```python
from build123d import *

# Parameters (mm, degrees)
SKETCH1_R           = 11.15
BOSS_EXTRUDE1_DEPTH = 15
FILLET3_R           = 0.8


with BuildPart() as part:
    # Sketch1 → Boss-Extrude1 (new body)
    with BuildSketch(Plane(origin=(0, 0, 0), x_dir=(1, 0, 0), z_dir=(0, 1, 0))):
        Polygon((0, 17.15), (2.145893606, 13.548639006), (5.299641454, 16.310619254), (6.227625801, 12.222403821), (10.080517077, 13.874641454), (9.699754592, 9.699754592), (13.874641454, 10.080517077), (12.222403821, 6.227625801), (16.310619254, 5.299641454), (13.548639006, 2.145893606), (17.15, 0), (13.548639006, -2.145893606), (16.310619254, -5.299641454), (12.222403821, -6.227625801), (13.874641454, -10.080517077), (9.699754592, -9.699754592), (10.080517077, -13.874641454), (6.227625801, -12.222403821), (5.299641454, -16.310619254), (2.145893606, -13.548639006), (0, -17.15), (-2.145893606, -13.548639006), (-5.299641454, -16.310619254), (-6.227625801, -12.222403821), (-10.080517077, -13.874641454), (-9.699754592, -9.699754592), (-13.874641454, -10.080517077), (-12.222403821, -6.227625801), (-16.310619254, -5.299641454), (-13.548639006, -2.145893606), (-17.15, 0), (-13.548639006, 2.145893606), (-16.310619254, 5.299641454), (-12.222403821, 6.227625801), (-13.874641454, 10.080517077), (-9.699754592, 9.699754592), (-10.080517077, 13.874641454), (-6.227625801, 12.222403821), (-5.299641454, 16.310619254), (-2.145893606, 13.548639006), align=None)
        Circle(SKETCH1_R, mode=Mode.SUBTRACT)
    extrude(amount=BOSS_EXTRUDE1_DEPTH)

    # Fillet3
    fillet3_edges = [part.edges().sort_by_distance(p)[0] for p in [
        (0, 7.5, -17.15),
        (5.299641454, 7.5, -16.310619254),
        (10.080517077, 7.5, -13.874641454),
        (13.874641454, 7.5, -10.080517077),
        (16.310619254, 7.5, -5.299641454),
        (17.15, 7.5, 0),
        (16.310619254, 7.5, 5.299641454),
        (13.874641454, 7.5, 10.080517077),
        (10.080517077, 7.5, 13.874641454),
        (5.299641454, 7.5, 16.310619254),
        (0, 7.5, 17.15),
        (-5.299641454, 7.5, 16.310619254),
        (-10.080517077, 7.5, 13.874641454),
        (-13.874641454, 7.5, 10.080517077),
        (-16.310619254, 7.5, 5.299641454),
        (-17.15, 7.5, 0),
        (-16.310619254, 7.5, -5.299641454),
        (-13.874641454, 7.5, -10.080517077),
        (-10.080517077, 7.5, -13.874641454),
        (-5.299641454, 7.5, -16.310619254),
    ]]
    fillet(fillet3_edges, radius=FILLET3_R)


solid = part.part
```
Geometry check sheet. Reference: the model listing, model coordinates, mm. A direction names the side the tool comes from. Give positions to 0.01 mm unless a question says otherwise; leave off trailing zeros. Write each loop counter-clockwise with the first axis right and the second up, starting at its lowest first coordinate (ties: lowest second). Pieces come first, ordered by that corner, then holes.
1) Access from +Z, -Z, +X, -X, +Y, -Y to the whole of each face (thin tool, end or side, straight path). Record for faces 5 (the flat face through (-14.8, 7.4, -1.4)), 6 (the flat face through (-1.4, 7.4, 14.8)), 7 (the flat face through (5.91, 7.4, -13.63)), 8 (the flat face through (14.8, 7.4, -1.4)).
2) Section check A-A, the plane z = 0. Record the boundary of the cut face in (x, y), and give its area (3 significant figures).
3) Gauge pin test, flat ends, axial feed: pin 1 (1 mm diameter, centred on y = 12.5, z = 3.5, fed in from -X); pin 2 (6 mm diameter, centred on y = 10, z = -9.5, fed in from -X); pin 3 (6 mm diameter, centred on y = 1.5, z = 3, fed in from +X); pin 4 (2 mm diameter, centred on y = 7, z = 9.5, fed in from +X). Record the tip position at first contact, or that the pin passes through.
4) Release check for a two-part mould opening along X. For faces 1 (the flat face through (-14.5, 7.4, 3.23)), 2 (the cylindrical face through (0.012, 7.605, 16.387)), 3 (the flat face through (13.63, 7.4, 5.91)), 4 (the cylindrical face through (10.635, 7.395, -3.349)) record: pulls with the +X half, pulls with the -X half, needs draft (parallel to the pull), parting line crosses it, or undercut.
5) Section check B-B, the plane x = 0. Record the boundary of the cut face in (y, z).
6) Material ranges on L1, parallel to Z at x = 0, y = 8.5; L2, parallel to X at y = 5.25, z = 14.5, recorded low to high.
Computed:
1. face 5: -X, +Y, -Y
1. face 6: +Z, +Y, -Y
1. face 7: -Z, +Y, -Y
1. face 8: +X, +Y, -Y
2. outline: (-16.39, 0) - (-11.15, 0) - (-11.15, 15) - (-16.39, 15) - close; (11.15, 0) - (16.39, 0) - (16.39, 15) - (11.15, 15) - close
2. area: 157 mm2
3. pin 1: stops at x = -15.17
3. pin 2: stops at x = -13.41
3. pin 3: stops at x = 16.39
3. pin 4: stops at x = 13.41
4. face 1: pulls with the -X half
4. face 2: parting line crosses it
4. face 3: pulls with the +X half
4. face 4: undercut
5. outline: (0, -16.39) - (15, -16.39) - (15, -11.15) - (0, -11.15) - close; (0, 11.15) - (15, 11.15) - (15, 16.39) - (0, 16.39) - close
6. L1: z = -16.39 to -11.15, 11.15 to 16.39
6. L2: x = -5.71 to -3.23, -1.58 to 1.58, 3.23 to 5.71
